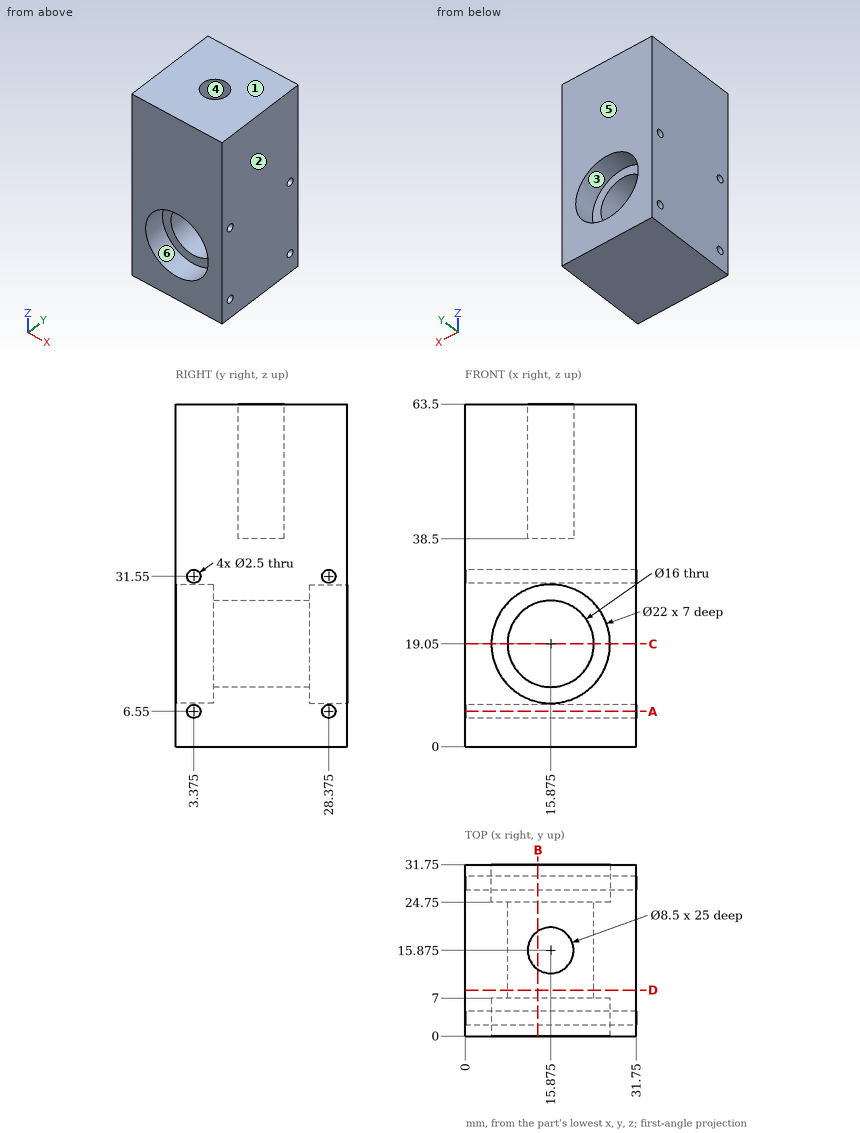
Study the drawing (mm; zero at the part's minimum x, y, z) and answer. A direction names the side the tool comes from. Give positions to 0.01 mm unless a question says otherwise; leave off trailing zeros. Write each loop counter-clockwise with the first axis right and the second up, starting at its lowest first coordinate (ties: lowest second). Pieces come first, ordered by that corner, then holes. Notation, with made-up numbers: (53, 35.5) - (70, 35.5) arc R25 ccw to (70, 69.5) - close; hole circle Ø1 at (65, 17.5). An arc over 180 degrees is marked (long way). Write item = value, one per line. Start each with the question number.
Item 1: Find section D-D (y = 8.5). Give the vertices of the cut face in (x, z) (3 decimals), then the cut area to 3 significant figures.
Item 2: The mould has two halves that part along X. Classify the marked faces 1, 2 and 3: +X half, -X half, draft (parallel to the pull), parting line (faces both ways), or undercut.
Item 3: Find the intervals of material crossed by probe 1 along X at (y, z) = (30, 19); probe 2 along X at (y, z) = (16, 50.5); probe 3 along Z at (x, y) = (14, 28), in increasing order. Write a range as [from, to].
Item 4: Find section B-B (x = 13.5). Give the vertices of the cut face in (y, z) (3 decimals), then the cut area to 3 significant figures.
Item 5: A tool of negligible diameter and unlimited length cuts with its end or side. For the marked faces 4, 5 and 6, from which of +Z, -Z, +X, -X, +Y, -Y can it reach the whole face along a straight path? Write none if from no direction.
Item 6: Each of these flat-tipped pins is pushed along its axis until it touches: P1, Ø6.5, axis at x = 10.5, z = 14, coming from the +Y side; P2, Ø2, axis at y = 28.375, z = 31.55, coming from the +X side; P3, Ø4, axis at x = 16, y = 14.5, coming from the +Z side. Where does it stop, or does it pass through?
Item 7: Find section C-C (z = 19.05). Give the vertices of the cut face in (x, y) (3 decimals), then the cut area to 3 significant figures.
Item 8: Find section A-A (z = 6.55). Give the vertices of the cut face in (x, y) (3 decimals), then the cut area to 3 significant figures.
Response:
q1.outline = (0, 0) - (31.75, 0) - (31.75, 63.5) - (0, 63.5) - close; hole circle Ø16 at (15.875, 19.05)
q1.area = 1,820 mm²
q2.face_1 = draft
q2.face_2 = +X half
q2.face_3 = undercut
q3.probe_1 = [0, 4.88], [26.87, 31.75]
q3.probe_2 = [0, 11.63], [20.12, 31.75]
q3.probe_3 = [0, 5.36], [7.74, 8.21], [29.89, 30.36], [32.74, 63.5]
q4.outline = (0, 0) - (31.75, 0) - (31.75, 8.309) - (24.75, 8.309) - (24.75, 11.411) - (7, 11.411) - (7, 8.309) - (0, 8.309) - close; (0, 29.791) - (7, 29.791) - (7, 26.689) - (24.75, 26.689) - (24.75, 29.791) - (31.75, 29.791) - (31.75, 63.5) - (19.399, 63.5) - (19.399, 38.5) - (12.351, 38.5) - (12.351, 63.5) - (0, 63.5) - close; hole circle Ø2.5 at (3.375, 6.55); hole circle Ø2.5 at (3.375, 31.55); hole circle Ø2.5 at (28.375, 6.55); hole circle Ø2.5 at (28.375, 31.55)
q4.area = 1,250 mm²
q5.face_4 = +Z
q5.face_5 = +Z, -Z, +X, -X, +Y
q5.face_6 = -Y
q6.P1 = 24.75
q6.P2 = through
q6.P3 = 38.5
q7.outline = (0, 0) - (4.875, 0) - (4.875, 7) - (7.875, 7) - (7.875, 24.75) - (4.875, 24.75) - (4.875, 31.75) - (0, 31.75) - close; (23.875, 7) - (26.875, 7) - (26.875, 0) - (31.75, 0) - (31.75, 31.75) - (26.875, 31.75) - (26.875, 24.75) - (23.875, 24.75) - close
q7.area = 416 mm²
q8.outline = (0, 0) - (31.75, 0) - (31.75, 2.125) - (0, 2.125) - close; (0, 4.625) - (31.75, 4.625) - (31.75, 27.125) - (0, 27.125) - close; (0, 29.625) - (31.75, 29.625) - (31.75, 31.75) - (0, 31.75) - close
q8.area = 849 mm²
